Autodesk Inventor part; units mm, degrees
ref_plane "YZ Plane" through (0, 0, 0) normal (1, 0, 0) x (0, 1, 0)
ref_plane "XZ Plane" through (0, 0, 0) normal (0, 1, 0) x (-1, 0, 0)
ref_plane "XY Plane" through (0, 0, 0) normal (0, 0, 1) x (1, 0, 0)
sketch "Sketch1" plane through (0, 0, 0) normal (0, 0, 1) x (1, 0, 0)
  line L0 (0, 2.3825) -> (0, -2.3825)
  line L1 (-5.7785, 0) -> (5.7785, 0)
  line L2 (4.1275, -1.7018) -> (-4.1275, -1.7018)
  line L3 (-4.1275, -1.7018) -> (-4.1275, 1.7018)
  line L4 (-4.1275, 1.7018) -> (4.1275, 1.7018)
  line L5 (4.1275, 1.7018) -> (4.1275, -1.7018)
  line L6 (4.1275, -1.7018) -> (-4.1275, 1.7018) construction
  line L7 (-4.1275, -1.7018) -> (4.1275, 1.7018) construction
  point P0 (0, 0)
  dimension "d0" = 8.255
  dimension "d1" = 3.4036
extrude "Extrusion1" add sketch "Sketch1" along normal blind 1.2192
sketch "Sketch2" plane through (4.1275, -1.7018, 0) normal (1, 0, 0) x (0, 0, -1)
  line L0 (0, 0) -> (-1.2192, 0)
  line L1 (-1.2192, 0) -> (-1.2192, 3.4036)
  line L2 (0, 3.4036) -> (0, 0)
  line L3 (-0.4572, 0) -> (-0.4572, 1.0033)
  line L4 (-0.4572, 1.0033) -> (-1.2192, 0.5634)
  line L5 (-1.2192, 0.5634) -> (-1.2192, 0)
  line L6 (-1.2192, 0) -> (-0.4572, 0)
  line L7 (-1.463, 1.7018) -> (0.2438, 1.7018)
  point P0 (0, 1.7018)
  dimension "d6" = 60
  dimension "d15" = 0.5634
  dimension "d28" = 0.6985
  dimension "d32" = 1.1384
  dimension "d33" = 0.4572
extrude "Extrusion2" cut sketch "Sketch2" against normal blind 8.255 contours L0 L1 L4 L3
mirror "Mirror1" about plane through (0, 0, 0) normal (0, 1, 0) of "Extrusion2"
sketch "Sketch5" plane through (-4.1275, 0, 0) normal (1, 0, 0) x (0, 1, 0)
  line L0 (1.7018, 0) -> (-1.7018, 0)
  line L1 (-1.7018, 0) -> (-1.7018, 0.4572)
  line L2 (1.7018, 0) -> (1.7018, 0.4572)
  line L3 (-1.7018, 0) -> (-2.0828, 0)
  line L4 (-2.0828, 0) -> (-2.0828, -0.3048)
  line L5 (-2.0828, -0.3048) -> (-1.7018, -0.3048)
  line L6 (-1.7018, -0.3048) -> (-1.7018, 0)
  line L7 (1.7018, 0) -> (2.0828, 0)
  line L8 (2.0828, 0) -> (2.0828, -0.3048)
  line L9 (2.0828, -0.3048) -> (1.7018, -0.3048)
  line L10 (1.7018, -0.3048) -> (1.7018, 0)
  line L11 (0, 1.524) -> (0, -0.6096)
  line L12 (-1.7018, 0.4572) -> (-2.0828, 0.4572)
  line L13 (-2.0828, 0.4572) -> (-2.0828, 0)
  point P0 (0, 0)
  dimension "d20" = 0.3048
  dimension "d29" = 0.381
extrude "Extrusion5" add sketch "Sketch5" along normal up to surface (8.255 mm away) contours L3 L13 L12 L1
extrude "Extrusion7" add sketch "Sketch5" along normal blind 4.826 contours L6 L5 L4 L3
properties part number "J008039 NEUROPIXELS DOVE TAIL MOUNT GEN 2 Rev -" material "ALUMINUM, 6061-T651"
Geometry check sheet. Reference: the model listing, model coordinates, mm. A direction names the side the tool comes from. Give positions to 0.01 mm unless a question says otherwise; leave off trailing zeros. Order: outer loops, then holes, each group sorted by start corner. A loop starts at its lowest first (then second) coordinate and runs counter-clockwise, first axis right, second up.
1. Section check A-A, the plane x = 2.25. Enter the section's corners in (y, z).
2. Section check B-B, the plane y = 1. Enter the section's corners in (x, z), and give its area (3 significant figures).
3. Thickness scan on L1, parallel to Z at x = -1.75, y = 0.05; L2, parallel to Z at x = 1, y = -0.9; L3, parallel to Z at x = -3.5, y = 0.95. Record the ranges inside material, lowest first.
4. Section check C-C, the plane x = -2.5. Enter the section's corners in (y, z), and give its area (3 significant figures).
5. Access from +Z, -Z, +X, -X, +Y, -Y to the whole of each face (thin tool, end or side, straight path). Record for faces 4 (the face through (-4.128, -0.2, 0.5)), 5 (the face through (0, -1, 0.457)).
6. Section check D-D, the plane y = -0.2. Enter the section's corners in (x, z).
7. Release check for a two-part mould opening along Z. For faces 1 (the face through (4.128, -0.2, 0.5)), 2 (the face through (0, 1, 0.457)), 3 (the face through (0, 0, 1.219)) record: pulls with the +Z half, pulls with the -Z half, needs draft (parallel to the pull), parting line crosses it, or undercut.
Values follow:
1. outline: (-2.08, 0) - (1.7, 0) - (1.7, 0.46) - (0.7, 0.46) - (1.14, 1.22) - (-1.14, 1.22) - (-0.7, 0.46) - (-2.08, 0.46) - close
2. outline: (-4.13, 0) - (4.13, 0) - (4.13, 0.46) - (-4.13, 0.46) - close; (-4.13, 0.98) - (4.13, 0.98) - (4.13, 1.22) - (-4.13, 1.22) - close
2. area: 5.75 mm2
3. L1: z = 0 to 1.22
3. L2: z = 0 to 0.46, 0.81 to 1.22
3. L3: z = 0 to 0.46, 0.89 to 1.22
4. outline: (-2.08, -0.3) - (-1.7, -0.3) - (-1.7, 0) - (1.7, 0) - (1.7, 0.46) - (0.7, 0.46) - (1.14, 1.22) - (-1.14, 1.22) - (-0.7, 0.46) - (-2.08, 0.46) - close
4. area: 3.25 mm2
5. face 4: +Z, -Z, -X, +Y, -Y
5. face 5: +X, -X, -Y
6. outline: (-4.13, 0) - (4.13, 0) - (4.13, 1.22) - (-4.13, 1.22) - close
7. face 1: needs draft
7. face 2: undercut
7. face 3: pulls with the +Z half
